Geometry: see drawing. Coordinates: mm, zero at the bounding-box minimum. Round coordinates to 2 decimals unless told otherwise and drop trailing zeros. Order: outer loops, then holes, each group sorted by start corner. A loop starts at its lowest first (then second) coordinate and runs counter-clockwise, first axis right, second up. Notation, with made-up numbers: (-1.5, -36.5) -> (12.5, -36.5) arc R16 cw to (12.5, -18.5) -> close; hole circle Ø6 at (23.25, 39). An arc over 180 degrees is marked (long way). Use a Markdown table: item, result.
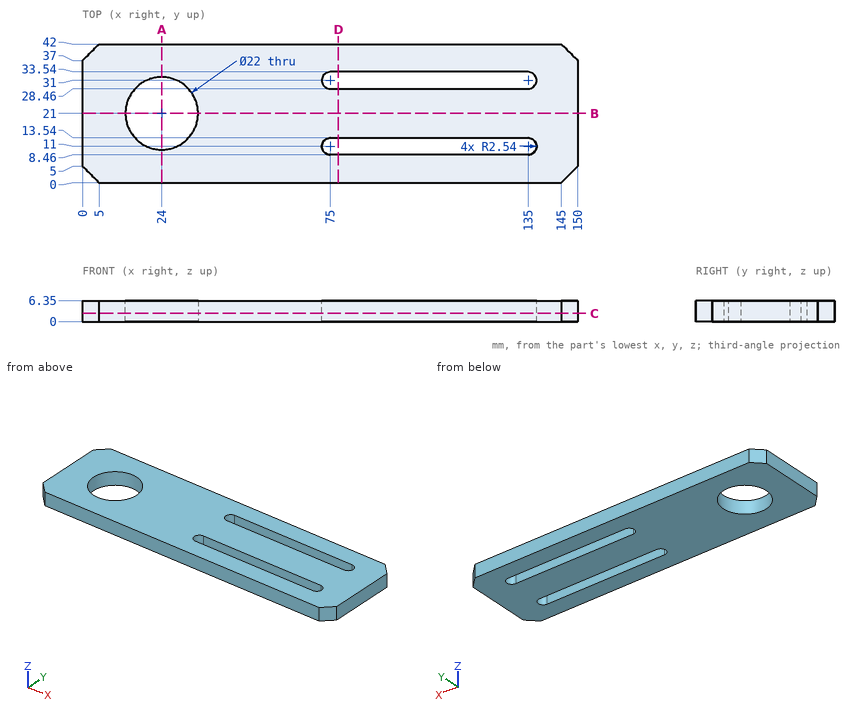
1) Cut plane D-D on x = 77.5. Return loops of the section in (y, z), and give its area (3 significant figures).
Answer key:
| item | result |
|---|---|
| outline | (0, 0) -> (8.46, 0) -> (8.46, 6.35) -> (0, 6.35) -> close; (13.54, 0) -> (28.46, 0) -> (28.46, 6.35) -> (13.54, 6.35) -> close; (33.54, 0) -> (42, 0) -> (42, 6.35) -> (33.54, 6.35) -> close |
| area | 202 mm^2 |
2) Ray query, probe 1 along Y at (x, z) = (82.5, 3.75); probe 2 along Y at (x, z) = (24, 5); probe 3 along X at (y, z) = (31, 1.5). Return the intervals inside material, ascending.
Answer key:
| item | result |
|---|---|
| probe 1 | y = 0 to 8.46, 13.54 to 28.46, 33.54 to 42 |
| probe 2 | y = 0 to 10, 32 to 42 |
| probe 3 | x = 0 to 19.42, 28.58 to 72.46, 137.54 to 150 |
3) Contact query for a flat-ended pin moving along its axis: P1, Ø20, axis at x = 24, y = 21, coming from the +Z side. Output: stop coordinate, or through.
Answer key:
| item | result |
|---|---|
| P1 | passes through |
4) Cut plane B-B on y = 21. Return loops of the section in (x, z).
Answer key:
| item | result |
|---|---|
| outline | (0, 0) -> (13, 0) -> (13, 6.35) -> (0, 6.35) -> close; (35, 0) -> (150, 0) -> (150, 6.35) -> (35, 6.35) -> close |
5) Cut plane A-A on x = 24. Return loops of the section in (y, z), and give its area (3 significant figures).
Answer key:
| item | result |
|---|---|
| outline | (0, 0) -> (10, 0) -> (10, 6.35) -> (0, 6.35) -> close; (32, 0) -> (42, 0) -> (42, 6.35) -> (32, 6.35) -> close |
| area | 127 mm^2 |
6) Cut plane C-C on z = 2.5. Return loops of the section in (x, y).
Answer key:
| item | result |
|---|---|
| outline | (0, 5) -> (5, 0) -> (145, 0) -> (150, 5) -> (150, 37) -> (145, 42) -> (5, 42) -> (0, 37) -> close; hole circle Ø22 at (24, 21); hole (75, 8.46) -> (135, 8.46) arc R2.54 ccw to (135, 13.54) -> (75, 13.54) arc R2.54 ccw to start; hole (75, 28.46) -> (135, 28.46) arc R2.54 ccw to (135, 33.54) -> (75, 33.54) arc R2.54 ccw to start |
